Design review of the part shown in the three views and the two pictorial views. Dimensions are in mm from the part's minimum x, y and z. Coordinates: 2 decimals unless noted, no trailing zeros. Loops run counter-clockwise (first coordinate to the right, second up) from the corner with the lowest first, then second, coordinate; pieces in that order, holes last. Notation, with made-up numbers: (14, -28) -> (69, -28) arc R37 cw to (69, 8) -> close; hole circle Ø10 at (12.25, 69.5). An arc over 180 degrees is marked (long way). Use a Markdown table: item, result. Add a question column.
Q1. For probe 1 along X at (y, z) = (1.85, 1.7) (1 decimal); probe 2 along Z at (x, y) = (2.75, 1.6); probe 3 along X at (y, z) = (1.5, 1.4) (1 decimal), list the stretches that pass through material, from the lowest coordinate up.
Q2. Clearance check with a flat-ended pin moving along its axis: pin 1 Ø1 at (x, y) = (5.5, 1.5) entering from +Z. State where the tip first meets the part, or that it passes through.
Q3. Draft analysis for pull direction X (two halves, no side actions). For the marked faces 1, 2, 3 and 4, state which applies: pulls with the +X half, pulls with the -X half, needs draft (parallel to the pull), parting line crosses it, or undercut.
Q4. Take a section at B-B on x = 5.5. Write out the cut boundary in (y, z).
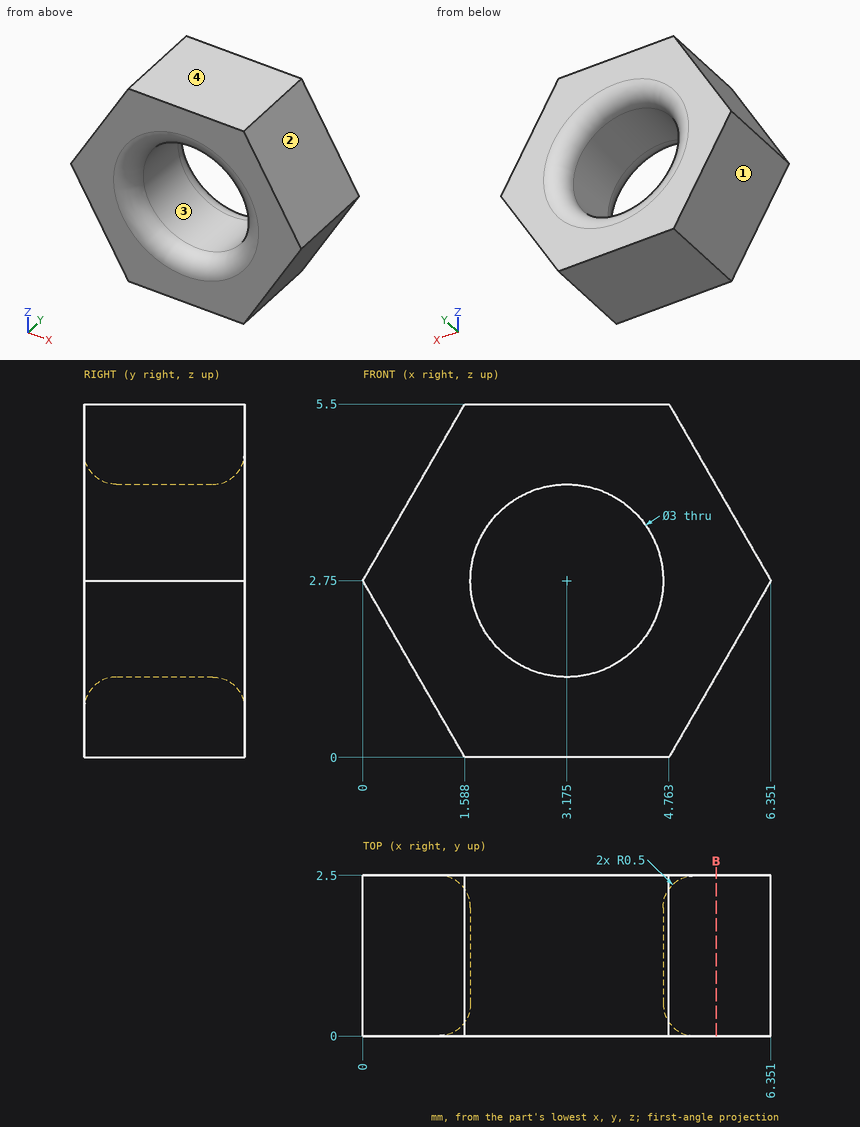
Answer list:
| question | item | result |
|---|---|---|
| 1 | probe 1 | 0.6 to 2.1, 4.2 to 5.7 |
| 1 | probe 2 | 0 to 1.31, 4.19 to 5.5 |
| 1 | probe 3 | 0.8 to 2.5, 3.8 to 5.6 |
| 2 | pin 1 | z = 5.09 |
| 3 | face 1 | pulls with the -X half |
| 3 | face 2 | pulls with the +X half |
| 3 | face 3 | undercut |
| 3 | face 4 | needs draft |
| 4 | outline | (0, 1.28) -> (2.5, 1.28) -> (2.5, 4.22) -> (0, 4.22) -> close |
